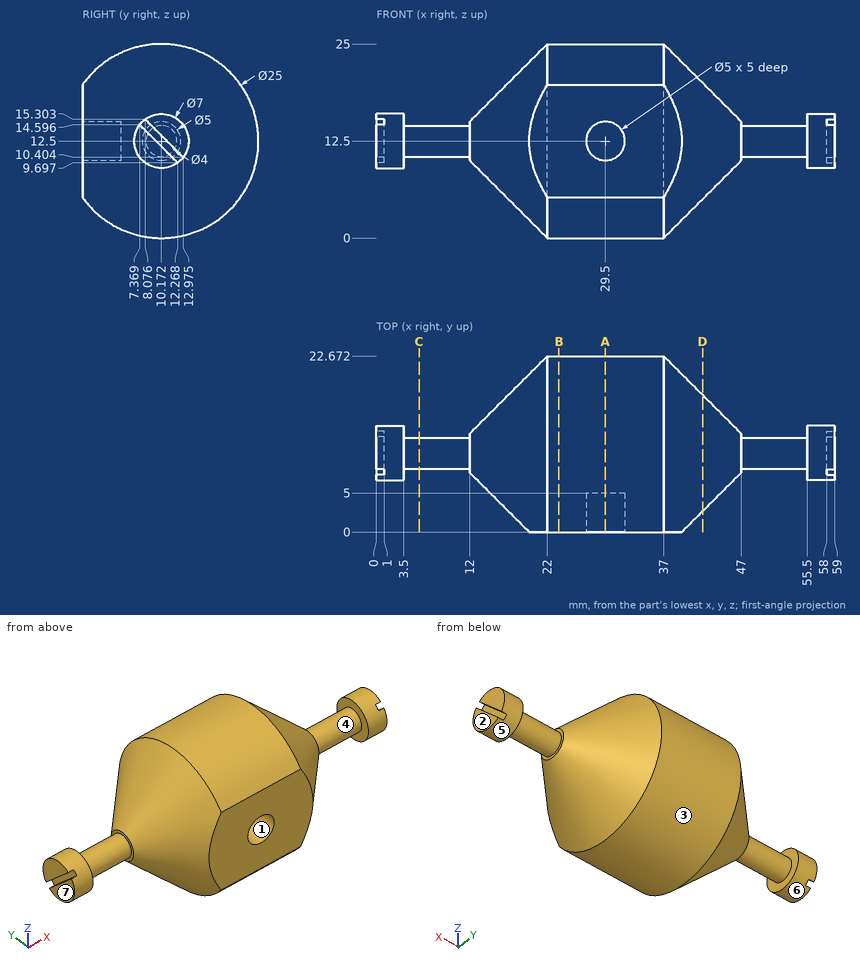
Source: three-view drawing plus pictorial views. Frame: mm from the lowest corner of the part. A direction names the side the tool comes from. Coordinates: 2 decimals unless noted, no trailing zeros. Order: outer loops, then holes, each group sorted by start corner. A loop starts at its lowest first (then second) coordinate and runs counter-clockwise, first axis right, second up.
1) Set-up query: the marked faces 4, 5, 6 and 7. Return all of +Z, -Z, +X, -X, +Y, -Y with unobstructed straight access to the full face (end or side cutting, diameter ignored); none if empty.
Result sheet:
face 4: none
face 5: +X
face 6: -X
face 7: +Z, -Z, -X, +Y, -Y
2) Ray query, probe 1 along X at (y, z) = (13, 11); probe 2 along X at (y, z) = (2.7, 12.5); probe 3 along X at (y, z) = (2.1, 12.5). Return the intervals inside material, ascending.
Result sheet:
probe 1: x = 0 to 3.5, 12.7 to 46.3, 55.5 to 59
probe 2: x = 16.97 to 27, 32 to 42.03
probe 3: x = 17.57 to 27, 32 to 41.43
3) Section B-B (x = 23.5). Return loops of the section in (y, z) (3 decimals).
Result sheet:
outline: (0, 5.235) arc R12.5 ccw (long way) to (0, 19.765) - close
4) Section D-D (x = 42). Return loops of the section in (y, z).
Result sheet:
outline: circle Ø15 at (10.17, 12.5)
5) First-contact query: P1, Ø12, axis at x = 8, y = 7.5, coming from the -Z side; P2, Ø1.5, axis at x = 29.5, z = 12, coming from the -Y side; P3, Ø3, axis at x = 18.5, z = 16.5, coming from the +Y side. Flat tips, straight axial feed; report the tip coordinate or a pass-through.
Result sheet:
P1: stops at z = 8.35
P2: stops at y = 5
P3: stops at y = 19.98
6) Draft query along X for the marked faces 1, 2 and 3. Return one class per face: released by +X, released by -X, zero draft, split by the parting line, or undercut.
Result sheet:
face 1: undercut
face 2: released by +X
face 3: zero draft
7) Section C-C (x = 5.5). Return loops of the section in (y, z).
Result sheet:
outline: circle Ø4 at (10.17, 12.5)
8) Section A-A (x = 29.5). Return loops of the section in (y, z) (3 decimals), then the cut area to 3 significant figures.
Result sheet:
outline: (0, 5.235) arc R12.5 ccw (long way) to (0, 19.765) - (0, 15) - (5, 15) - (5, 10) - (0, 10) - close
area: 443 mm2
